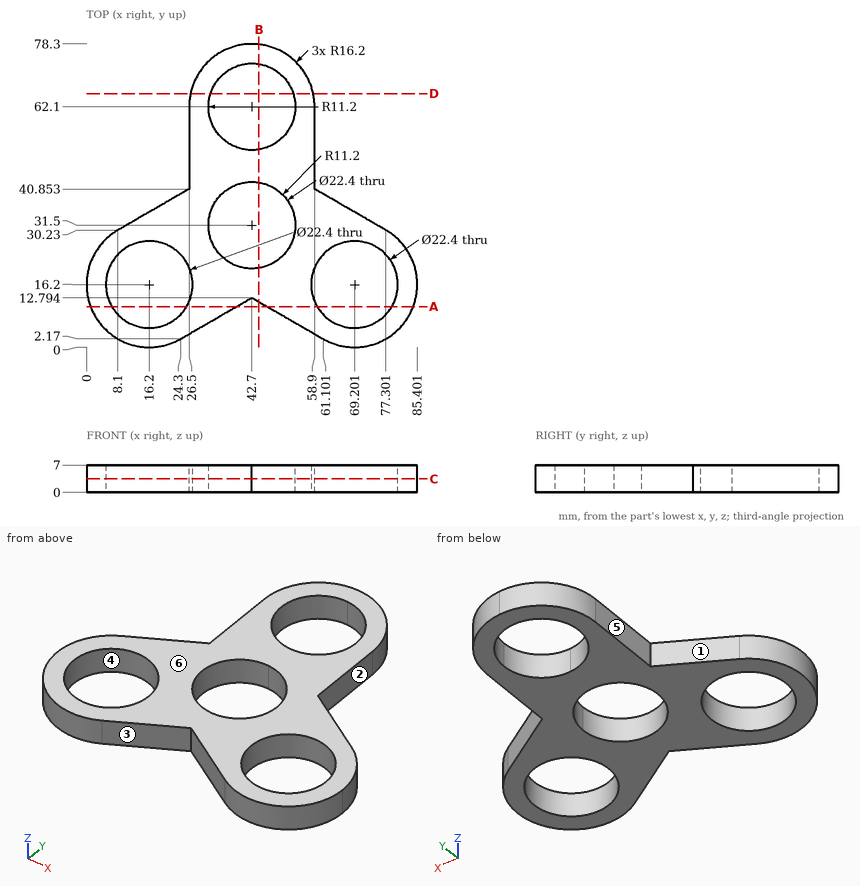
Input: dimensioned drawing with shaded views. Units: mm. Origin: part minimum x, y, z. A direction names the side the tool comes from. Round coordinates to 2 decimals unless told otherwise and drop trailing zeros. Loops run counter-clockwise (first coordinate to the right, second up) from the corner with the lowest first, then second, coordinate; pieces in that order, holes last. Notation, with made-up numbers: (29.5, 0.25) -> (78.5, 0.25) arc R22 ccw to (78.5, 19.25) -> close; hole circle Ø4 at (-12, 43). An arc over 180 degrees is marked (long way). Answer as a JSON object with one key per item and string values. Group by question number.
Q1. Access query for the marked faces 1, 2 and 3. Directions: +Z, -Z, +X, -X, +Y, -Y. A direction counts if a zero-diameter tool reaches every point of the face in a straight line with its end or side. Return the directions, or none.
Q2. Section query A-A (y = 10.5). Output: boundary loops of the cut face in (x, z) (1 decimal).
Q3. Section query D-D (y = 65.5). Output: boundary loops of the cut face in (x, z).
Q4. Ray query, line 1 (X direction, y = 16.2, z = 2.75); line 2 (X direction, y = 11.5, z = 6.5) (1 decimal); line 3 (X direction, y = 11, z = 3.5) (1 decimal). Return the intervals inside material, ascending. Write a range as from..to.
Q5. Section query C-C (z = 3.5). Output: boundary loops of the cut face in (x, y), plus the area to 3 significant figures.
Q6. Contact query for flat-ended pins moving along their axis: P1, Ø1, axis at x = 17, z = 4.5, coming from the -Y side; P2, Ø1, axis at y = 60, z = 2, coming from the -X side; P3, Ø2, axis at x = 74.5, z = 3.5, coming from the -Y side. Output: stop coordinate, or through.
Q7. Section query B-B (x = 44.5). Output: boundary loops of the cut face in (y, z) (1 decimal).
Q8. Mould query, pull axis X, two halves, no side actions, for the marked faces 4, 5 and 6. Classes: pulls with the +X half, pulls with the -X half, needs draft (parallel to the pull), parting line crosses it, or undercut.
Completed:
{
 "1": {"face 1": "+Z, -Z, -X, +Y", "face 2": "+Z, -Z, +X, +Y", "face 3": "+Z, -Z, -Y"},
 "2": {"outline": "(1, 0) -> (6.6, 0) -> (6.6, 7) -> (1, 7) -> close; (25.8, 0) -> (38.7, 0) -> (38.7, 7) -> (25.8, 7) -> close; (46.7, 0) -> (59.6, 0) -> (59.6, 7) -> (46.7, 7) -> close; (78.8, 0) -> (84.4, 0) -> (84.4, 7) -> (78.8, 7) -> close"},
 "3": {"outline": "(26.86, 0) -> (32.03, 0) -> (32.03, 7) -> (26.86, 7) -> close; (53.37, 0) -> (58.54, 0) -> (58.54, 7) -> (53.37, 7) -> close"},
 "4": {"line 1": "0..5, 27.4..58, 80.4..85.4", "line 2": "0.7..6, 26.4..40.5, 44.9..59, 79.4..84.7", "line 3": "0.9..6.3, 26.1..39.6, 45.8..59.3, 79.1..84.5"},
 "5": {"outline": "(8.1, 30.23) arc R16.2 ccw to (24.3, 2.17) -> (42.7, 12.79) -> (61.1, 2.17) arc R16.2 ccw to (77.3, 30.23) -> (58.9, 40.85) -> (58.9, 62.1) arc R16.2 ccw to (26.5, 62.1) -> (26.5, 40.85) -> close; hole circle Ø22.4 at (16.2, 16.2); hole circle Ø22.4 at (42.7, 31.5); hole circle Ø22.4 at (42.7, 62.1); hole circle Ø22.4 at (69.2, 16.2)", "area": "2,180 mm²"},
 "6": {"P1": "y = 0", "P2": "x = 26.5", "P3": "y = 0.58"},
 "7": {"outline": "(11.8, 0) -> (20.4, 0) -> (20.4, 7) -> (11.8, 7) -> close; (42.6, 0) -> (51, 0) -> (51, 7) -> (42.6, 7) -> close; (73.2, 0) -> (78.2, 0) -> (78.2, 7) -> (73.2, 7) -> close"},
 "8": {"face 4": "undercut", "face 5": "pulls with the -X half", "face 6": "needs draft"}
}
